Source: CAD feature listing. Evaluate the final solid. Frame: model axes, mm. Face numbers are marked on the shaded views. A direction names the side the tool comes from. Give positions to 0.01 mm unless a question says otherwise; leave off trailing zeros. Order: outer loops, then holes, each group sorted by start corner. A loop starts at its lowest first (then second) coordinate and runs counter-clockwise, first axis right, second up. Notation, with made-up numbers: (-1, 6) -> (25, 6) arc R29 ccw to (25, 33) -> close; hole circle Ø5 at (82.25, 62). An arc over 180 degrees is marked (long way). Use CSV: the item, a comma, the result in double quotes.
```python
from build123d import *

# Parameters (mm, degrees)
M3_5X0_6_TAPPED_HOLE1_D     = 2.9
M3_5X0_6_TAPPED_HOLE1_DEPTH = 4.064
M3_5X0_6_TAPPED_HOLE1_TIP   = 0.871247898


with BuildPart() as part:
    # Sketch1 → Revolve1 (revolve)
    with BuildSketch(Plane.XY, mode=Mode.PRIVATE) as revolve1_sk:
        Polygon((0, 30.65), (0, 0), (13.95, 0), (13.95, 2.54), (2.54, 5.08), (2.54, 5.95), (13.95, 5.95), (13.95, 18.65), (2.5, 18.65), (2.5, 30.65), align=None)
    revolve(revolve1_sk.sketch.rotate(Axis((0, 0, 0), (0, 1, 0)), 90), axis=Axis((0, 0, 0), (0, 1, 0)))

    # M3.5x0.6 Tapped Hole1
    with Locations(Plane(origin=(-5.656854249, 0, 5.656854249), x_dir=(0, 0, -1), z_dir=(0, -1, 0))):
        with Locations((0, 0), (0, 11.313708498), (11.313708498, 11.313708498), (11.313708498, 0)):
            Hole(M3_5X0_6_TAPPED_HOLE1_D / 2, depth=M3_5X0_6_TAPPED_HOLE1_DEPTH)
            with Locations((0, 0, -(M3_5X0_6_TAPPED_HOLE1_DEPTH + M3_5X0_6_TAPPED_HOLE1_TIP / 2))):  # 118° drill point
                Cone(0, M3_5X0_6_TAPPED_HOLE1_D / 2, M3_5X0_6_TAPPED_HOLE1_TIP, mode=Mode.SUBTRACT)


solid = part.part
```
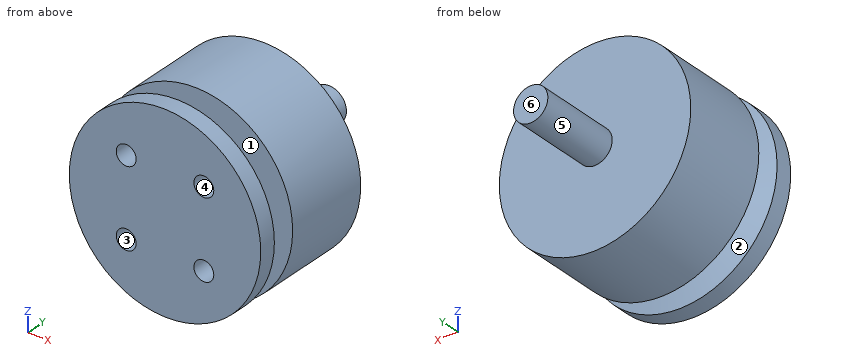
1. Access query for the marked faces 4, 5 and 6. Directions: +Z, -Z, +X, -X, +Y, -Y. A direction counts if a zero-diameter tool reaches every point of the face in a straight line with its end or side. Return the directions, or none.
Answer below:
face 4,"-Y"
face 5,"+Y"
face 6,"+Z, -Z, +X, -X, +Y"
2. Section query B-B on x = 0. Return loops of the section in (y, z), plus the area to 4 significant figures.
Answer below:
outline,"(0, -13.95) -> (2.54, -13.95) -> (5.08, -2.54) -> (5.95, -2.54) -> (5.95, -13.95) -> (18.65, -13.95) -> (18.65, -2.5) -> (30.65, -2.5) -> (30.65, 2.5) -> (18.65, 2.5) -> (18.65, 13.95) -> (5.95, 13.95) -> (5.95, 2.54) -> (5.08, 2.54) -> (2.54, 13.95) -> (0, 13.95) -> close"
area,"531.5 mm²"
3. Mould query, pull axis X, two halves, no side actions, for the marked faces 1, 2 and 3. Classes: released by +X, released by -X, zero draft, split by the parting line, or undercut.
Answer below:
face 1,"zero draft"
face 2,"split by the parting line"
face 3,"undercut"
4. Section query A-A on z = 0. Return loops of the section in (x, y), plus the area to 4 significant figures.
Answer below:
outline,"(-13.95, 0) -> (13.95, 0) -> (13.95, 2.54) -> (2.54, 5.08) -> (2.54, 5.95) -> (13.95, 5.95) -> (13.95, 18.65) -> (2.5, 18.65) -> (2.5, 30.65) -> (-2.5, 30.65) -> (-2.5, 18.65) -> (-13.95, 18.65) -> (-13.95, 5.95) -> (-2.54, 5.95) -> (-2.54, 5.08) -> (-13.95, 2.54) -> close"
area,"531.5 mm²"
5. Section query C-C on y = 20. Return loops of the section in (x, z).
Answer below:
outline,"circle Ø5 at (0, 0)"
6. Ray query, line 1 along Z through (x, y) = (0.5, 12.5); line 2 along X through (y, z) = (14, 0.25); line 3 along Y through (x, z) = (0.25, 12.75). Return the intervals inside material, ascending.
Answer below:
line 1,"z = -13.94 to 13.94"
line 2,"x = -13.95 to 13.95"
line 3,"y = 0 to 2.81, 5.95 to 18.65"
7. Section query D-D on z = 4.75. Count the separate pieces of the cut face and the enclosed holes in it, plus the area to 3 significant figures.
Answer below:
separate pieces,"4"
enclosed holes,"0"
area,"414 mm²"
8. Pin query (flat end, axial travel): P1, Ø1.5, axis at y = 15, z = 3.5, coming from the +X side; P2, Ø2.5, axis at x = -5.66, z = 5.66, coming from the -Y side; P3, Ø6, axis at x = 2.5, y = 20.5, coming from the +Z side. Return the tip coordinate at first contact, or that it passes through.
Answer below:
P1,"stops at x = 13.68"
P2,"stops at y = 5.95"
P3,"stops at z = 13.95"
